```python
from build123d import *

# Parameters (mm, degrees)
EXTRUDE_1_DEPTH             = 3
SKETCH_2_W                  = 243.8
SKETCH_2_H                  = 3
EXTRUDE_2_DEPTH             = 62.5
SKETCH_3_W                  = 79.68324927
SKETCH_3_H                  = 3
EXTRUDE_3_DEPTH             = 5
SKETCH_4_W                  = 79.68324927
SKETCH_4_H                  = 3
EXTRUDE_4_DEPTH             = 40
HOLE_WIZARD_2_5_2_5_1_D     = 2.5
HOLE_WIZARD_25_0_25_1_D     = 25
HOLE_WIZARD_25_0_25_1_DEPTH = 43
HOLE_WIZARD_M641_D          = 71.5
HOLE_WIZARD_M641_DEPTH      = 43
HOLE_WIZARD_3_4_3_4_1_D     = 3.4
HOLE_WIZARD_3_4_3_4_1_DEPTH = 43
HOLE_WIZARD_2_5_2_5_2_D     = 2.5
HOLE_WIZARD_2_5_2_5_2_DEPTH = 43
FILLET_1_R                  = 0.5
FILLET_2_R                  = 3
FILLET_3_R                  = 3.5
FILLET_4_R                  = 44.4


with BuildPart() as part:
    # Эскиз1 → Бобышка-Вытянуть1 (new body)
    with BuildSketch(Plane.XZ.offset(-247)):
        with BuildLine():
            Line((124.999894737, -9.1), (-124.999894737, -9.1))
            ThreePointArc((-124.999894737, -9.1), (-119.638879455, -30.921789121), (-104.847515108, -47.837654634))
            Line((-104.847515108, -47.837654634), (-41.341624635, -92.555295683))
            Line((-41.341624635, -92.555295683), (-41.341624635, -88.5))
            Line((-41.341624635, -88.5), (41.341624635, -88.5))
            Line((41.341624635, -88.5), (41.341624635, -92.555295631))
            Line((41.341624635, -92.555295631), (104.847515108, -47.837654582))
            ThreePointArc((104.847515108, -47.837654582), (119.638879443, -30.921789092), (124.999894737, -9.1))
        make_face()
    extrude(amount=-EXTRUDE_1_DEPTH)

    # Эскиз2 → Бобышка-Вытянуть2 (add)
    with BuildSketch(Plane.XY.offset(-9.1)):
        with Locations((2e-09, 248.5)):
            Rectangle(SKETCH_2_W, SKETCH_2_H)
    extrude(amount=EXTRUDE_2_DEPTH)

    # Эскиз3 → Бобышка-Вытянуть3 (add)
    with BuildSketch(Plane(origin=(0, 0, -88.5), x_dir=(-1, 0, 0), z_dir=(0, 0, -1))):
        with Locations((0, 248.5)):
            Rectangle(SKETCH_3_W, SKETCH_3_H)
    extrude(amount=EXTRUDE_3_DEPTH)

    # Эскиз4 → Бобышка-Вытянуть4 (add)
    with BuildSketch(Plane(origin=(0, 250, 0), x_dir=(-1, 0, 0), z_dir=(0, 1, 0))):
        with Locations((0, -92)):
            Rectangle(SKETCH_4_W, SKETCH_4_H)
    extrude(amount=EXTRUDE_4_DEPTH)

    # Диаметр отверстия Ø2.5 (2.5)1 (through all)
    with Locations(Plane.XY.offset(-90.5)):
        with Locations((25, 266), (25, 282), (0, 266), (0, 282), (-25, 266), (-25, 282)):
            Hole(HOLE_WIZARD_2_5_2_5_1_D / 2)

    # Диаметр отверстия Ø25.0 (25)1
    with Locations(Plane(origin=(0, 247, 0), x_dir=(-1, 0, 0), z_dir=(0, -1, 0))):
        with Locations((0, 60)):
            Hole(HOLE_WIZARD_25_0_25_1_D / 2, depth=HOLE_WIZARD_25_0_25_1_DEPTH)

    # Отверстие с зазором M641
    with Locations(Plane(origin=(0, 247, 0), x_dir=(-1, 0, 0), z_dir=(0, -1, 0))):
        with Locations((72, 0), (-72, 0)):
            Hole(HOLE_WIZARD_M641_D / 2, depth=HOLE_WIZARD_M641_DEPTH)

    # Диаметр отверстия Ø3.4 (3.4)1
    with Locations(Plane(origin=(0, 247, 0), x_dir=(-1, 0, 0), z_dir=(0, -1, 0))):
        with Locations((72, 41.5), (42.655068581, 29.344931419), (30.5, 0), (42.655068581, -29.344931419), (72, -41.5), (101.344931419, -29.344931419), (101.344931419, 29.344931419), (-101.344931419, 29.344931419), (-101.344931419, -29.344931419), (-72, -41.5), (-42.655068581, -29.344931419), (-30.5, 0), (-42.655068581, 29.344931419), (-72, 41.5)):
            Hole(HOLE_WIZARD_3_4_3_4_1_D / 2, depth=HOLE_WIZARD_3_4_3_4_1_DEPTH)

    # Диаметр отверстия Ø2.5 (2.5)2
    with Locations(Plane(origin=(0, 247, 0), x_dir=(-1, 0, 0), z_dir=(0, -1, 0))):
        with Locations((-20, 58.5), (20, 18.5), (-20, 18.5), (-20, -1.5), (20, -21.5), (20, -41.5), (-20, -41.5), (-20, -21.5), (20, -1.5), (-20, 38.5), (20, 38.5), (-40, 58.5), (-40, 78.5), (-20, 78.5), (20, 58.5), (20, 78.5), (40, 58.5), (40, 78.5)):
            Hole(HOLE_WIZARD_2_5_2_5_2_D / 2, depth=HOLE_WIZARD_2_5_2_5_2_DEPTH)

    # Скругление1
    fillet_1_edges = [part.edges().sort_by_distance(p)[0] for p in [
        (0, 250, -90.5),
    ]]
    fillet(fillet_1_edges, radius=FILLET_1_R)

    # Скругление2
    fillet_2_edges = [part.edges().sort_by_distance(p)[0] for p in [
        (-39.841624635, 290, -92),
        (39.841624635, 290, -92),
    ]]
    fillet(fillet_2_edges, radius=FILLET_2_R)

    # Скругление3
    fillet_3_edges = [part.edges().sort_by_distance(p)[0] for p in [
        (0, 247, -93.5),
    ]]
    fillet(fillet_3_edges, radius=FILLET_3_R)

    # Скругление4
    fillet_4_edges = [part.edges().sort_by_distance(p)[0] for p in [
        (121.900000002, 248.5, 53.4),
        (-121.899999998, 248.5, 53.4),
    ]]
    fillet(fillet_4_edges, radius=FILLET_4_R)


solid = part.part
```
Could you check a few things on this model? Use its own coordinates, in mm. A direction names the side the tool comes from. Coordinates: 2 decimals unless noted, no trailing zeros. Loops run counter-clockwise (first coordinate to the right, second up) from the corner with the lowest first, then second, coordinate; pieces in that order, holes last.
1) Imagine slicing it at C-C (x = 55.5). List the corners of the cut face in (y, z) for me.
Reported:
outline: (247, -82.59) - (250, -82.59) - (250, -31.71) - (247, -31.71) - close; (247, 31.71) - (250, 31.71) - (250, 53.4) - (247, 53.4) - close
2) Please list where these lines run through material, in increasing order: line 1 along X through (y, z) = (247.95, 41.5); line 2 along X through (y, z) = (249.25, -41.5); line 3 along Y through (x, z) = (-6.5, -83).
Reported:
line 1: x = -107.75 to -73.7, -70.3 to -21.25, -18.75 to 18.75, 21.25 to 70.3, 73.7 to 107.75
line 2: x = -112.14 to -73.7, -70.3 to 70.3, 73.7 to 112.14
line 3: y = 247 to 250
3) Will these pins go through, and if not, where does the flat tip stop? pin 1 Ø5 at (x, y) = (76, 252) entering from -Z; pin 2 Ø3 at (x, z) = (40, -58.5) entering from +Y; pin 3 Ø0.9 at (x, y) = (124, 249) entering from +Z.
Reported:
pin 1: stops at z = -69.21
pin 2: stops at y = 250
pin 3: stops at z = -9.1
4) Imagine slicing it at A-A (x = -90.5). List the corners of the cut face in (y, z) for me.
Reported:
outline: (247, -57.94) - (250, -57.94) - (250, -30.59) - (247, -30.59) - close; (247, 30.59) - (250, 30.59) - (250, 51.45) - (247, 51.45) - close
5) Thinking about a two-plate mould opening in Z: for faces 1 (the face through (109.24, 248.52, 40.05)), 2 (the face through (-37.9, 248.52, -10.74)), 3 (the face through (-73.539, 248.479, -69.883)), which applies, released by +Z, released by -Z, zero draft, split by the parting line, or undercut?
Reported:
face 1: released by +Z
face 2: undercut
face 3: released by -Z
6) Which directions (+Z, -Z, +X, -X, +Y, -Y) give clear straight access to the entire face, cutting with the end or side of a thin tool? Please do faces 4 (the face through (-39.842, 267, -92)), 5 (the face through (119.491, 248.479, -31.203)), 6 (the face through (1, 270, -90.5)).
Reported:
face 4: -Z, +Y, -Y
face 5: -Z, +X, +Y, -Y
face 6: +Z, +X, -X, +Y
7) Imagine slicing it at B-B (y = 255). List the corners of the cut face in (x, z) for me.
Reported:
outline: (-39.84, -93.5) - (39.84, -93.5) - (39.84, -90.5) - (-39.84, -90.5) - close
